```python
from build123d import *

# Parameters (mm, degrees)
BOSS_EXTRUDE1_DEPTH = 1.000000032
SKETCH2_W           = 4.49999989
SKETCH2_H           = 5.735208424
SKETCH2_W_2         = 3
SKETCH2_H_2         = 2
BOSS_EXTRUDE2_DEPTH = 1
SKETCH3_W           = 2.900000042
SKETCH3_H           = 8.000000002
BOSS_EXTRUDE3_DEPTH = 1.94999991


with BuildPart() as part:
    # Sketch1 → Boss-Extrude1 (new body)
    with BuildSketch(Plane(origin=(0, 0, 0), x_dir=(1, 0, 0), z_dir=(0, 1, 0))):
        Polygon((-3.499999985, 9.50000005), (-0.499999889, 12.500000146), (0.499999889, 12.500000146), (3.499999985, 9.50000005), (4.999999906, 9.50000005), (20.000000132, 9.50000005), (20.000000132, -9.50000005), (4.999999906, -9.50000005), (3.499999985, -9.50000005), (0.499999889, -12.500000146), (-0.499999889, -12.500000146), (-3.499999985, -9.50000005), (-4.999999906, -9.50000005), (-4.999999906, 9.50000005), align=None)
    extrude(amount=-BOSS_EXTRUDE1_DEPTH)

    # Sketch2 → Boss-Extrude2 (add)
    with BuildSketch(Plane(origin=(0, 0, 0), x_dir=(1, 0, 0), z_dir=(0, 1, 0))):
        Rectangle(SKETCH2_W, SKETCH2_H)
        with Locations((-1.5875, 5.842)):
            Rectangle(SKETCH2_W_2, SKETCH2_H_2)
    extrude(amount=BOSS_EXTRUDE2_DEPTH)

    # Sketch3 → Boss-Extrude3 (add)
    with BuildSketch(Plane(origin=(0, 0, 0), x_dir=(1, 0, 0), z_dir=(0, 1, 0))):
        with Locations((17.756250111, 0)):
            Rectangle(SKETCH3_W, SKETCH3_H)
    extrude(amount=BOSS_EXTRUDE3_DEPTH)


solid = part.part
```
Geometry: final body of the model. Coordinates: model frame, mm. A direction names the side the tool comes from. Coordinates: 2 decimals unless noted, no trailing zeros. Order: outer loops, then holes, each group sorted by start corner. A loop starts at its lowest first (then second) coordinate and runs counter-clockwise, first axis right, second up. Notation, with made-up numbers: (20, -37.5) -> (39, -37.5) arc R29 cw to (39, -16.5) -> close; hole circle Ø10 at (65, 70). An arc over 180 degrees is marked (long way). Write item = value, one per line.
(1) Access query for faces 1 (the flat face through (-0.087, 0.5, -5.8)), 2 (the flat face through (-1.6, 0.5, -6.842)), 3 (the flat face through (-4.2, -0.5, 9.5)), 4 (the flat face through (0, 0.5, 2.868)). Directions: +Z, -Z, +X, -X, +Y, -Y. A direction counts if a zero-diameter tool reaches every point of the face in a straight line with its end or side. Return the directions, or none.
Solved:
face_1 = -Z, +X, +Y
face_2 = -Z, +X, -X, +Y
face_3 = +Z, -X, +Y, -Y
face_4 = +Z, -X, +Y
(2) Line query: line 1 (Y direction, x = 4, z = 2.5); line 2 (Z direction, x = 16.75, y = 1); line 3 (Z direction, x = 2, y = 0.55). Output: solid intervals per line, ascending.
Solved:
line_1 = -1 to 0
line_2 = -4 to 4
line_3 = -2.87 to 2.87
(3) Cut plane D-D on z = 2.5. Return loops of the section in (x, y), plus the area to 3 significant figures.
Solved:
outline = (-5, -1) -> (20, -1) -> (20, 0) -> (19.21, 0) -> (19.21, 1.95) -> (16.31, 1.95) -> (16.31, 0) -> (2.25, 0) -> (2.25, 1) -> (-2.25, 1) -> (-2.25, 0) -> (-5, 0) -> close
area = 35.2 mm²
(4) Cut plane A-A on y = 0.55. Return loops of the section in (x, z).
Solved:
outline = (-3.09, -6.84) -> (-0.09, -6.84) -> (-0.09, -4.84) -> (-3.09, -4.84) -> close; (-2.25, -2.87) -> (2.25, -2.87) -> (2.25, 2.87) -> (-2.25, 2.87) -> close; (16.31, -4) -> (19.21, -4) -> (19.21, 4) -> (16.31, 4) -> close
(5) Pull-direction query (X, two-part tool) for faces 5 (the flat face through (18, 1, -4)), 6 (the flat face through (-3.088, 0.5, -5.8)), 7 (the flat face through (2, -0.5, -11)), 8 (the flat face through (8, 0, 0)); classes: pulls with the +X half, pulls with the -X half, needs draft (parallel to the pull), parting line crosses it, or undercut.
Solved:
face_5 = needs draft
face_6 = pulls with the -X half
face_7 = pulls with the +X half
face_8 = undercut
(6) Cut plane B-B on x = 1.5. Return loops of the section in (y, z).
Solved:
outline = (-1, -11.5) -> (0, -11.5) -> (0, -2.87) -> (1, -2.87) -> (1, 2.87) -> (0, 2.87) -> (0, 11.5) -> (-1, 11.5) -> close
(7) Pin query (flat end, axial travel): pin 1 Ø2 at (x, z) = (-0.5, -1) entering from +Y; pin 2 Ø0.5 at (y, z) = (0.5, 1) entering from +X; pin 3 Ø0.8 at (y, z) = (0.5, 0) entering from -X. Return the tip coordinate at first contact, or that it passes through.
Solved:
pin_1 = 1
pin_2 = 19.21
pin_3 = -2.25
(8) Cut plane C-C on z = -6. Return loops of the section in (x, y).
Solved:
outline = (-5, -1) -> (20, -1) -> (20, 0) -> (-0.09, 0) -> (-0.09, 1) -> (-3.09, 1) -> (-3.09, 0) -> (-5, 0) -> close
